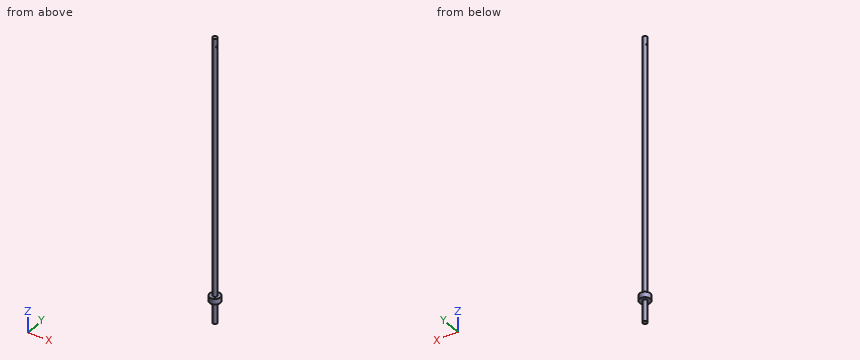
from build123d import *

# Parameters (mm, degrees)
F0_R     = 4
F1_DEPTH = 500
F3_START = -450
F2_R     = 10
F2_R_2   = 4
F3_DEPTH = 10
F4_DEPTH = 25
F5_R     = 2
F6_DEPTH = 12.5


with BuildPart() as f1:
    # F0 (on Top) → F1 (new body)
    with BuildSketch(Plane.XY):
        Circle(F0_R)
    extrude(amount=-F1_DEPTH)

    # F2 (on Top) → F3 (join)
    with BuildSketch(Plane.XY.offset(F3_START)):
        Circle(F2_R)
        Circle(F2_R_2, mode=Mode.SUBTRACT)
    extrude(amount=-F3_DEPTH)

    # F0 (on Top) → F4 (join)
    with BuildSketch(Plane.XY):
        Circle(F0_R)
    extrude(amount=F4_DEPTH)

    # F5 (on Right) → F6 (cut, symmetric)
    with BuildSketch(Plane.YZ):
        with Locations((0, 10)):
            Circle(F5_R)
    extrude(amount=F6_DEPTH, both=True, mode=Mode.SUBTRACT)


solid = f1.part
For this review, take the finished solid that the model builds, in its own axes (mm). Round coordinates to 2 decimals unless told otherwise and drop trailing zeros. Write each loop counter-clockwise with the first axis right and the second up, starting at its lowest first coordinate (ties: lowest second). Pieces come first, ordered by that corner, then holes. Notation, with made-up numbers: M 76,-28 L 99,-28 A24 ccw 99,3 Z; hole C 10,54 d4. An arc over 180 degrees is marked long. Write item = value, one per line. Start each with the question number.
(1) Clearance check with flat-ended pins moving along their axes: pin 1 Ø6 at (x, y) = (5.5, -5.5) entering from -Z; pin 2 Ø6 at (y, z) = (0.5, -315) entering from +X; pin 3 Ø1.5 at (x, y) = (1, 6.5) entering from +Z. State where each tip first meets the part, or that it passes through.
(2) We need section B-B (z = -230). Give the boundary of the cut face in (x, y), then the cut area to 3 significant figures.
(3) For line 1 along Z through (x, y) = (1, 0); line 2 along Y through (x, z) = (-0.25, 10); line 3 along Y through (x, z) = (-0.75, 10), list the stretches that pass through material, from the lowest coordinate up.
(4) We need section A-A (x = 0). Give the boundary of the cut face in (y, z).
Results found:
q1.pin_1 = -460
q1.pin_2 = 4
q1.pin_3 = -450
q2.outline = C 0,0 d8
q2.area = 50.3 mm²
q3.line_1 = -500 to 8, 12 to 25
q3.line_2 = -3.99 to -2, 2 to 3.99
q3.line_3 = -3.93 to -2, 2 to 3.93
q4.outline = M -10,-460 L -4,-460 L -4,-500 L 4,-500 L 4,-460 L 10,-460 L 10,-450 L 4,-450 L 4,25 L -4,25 L -4,-450 L -10,-450 Z; hole C 0,10 d4
